Part model, mm, in its own coordinate system. Face numbers are marked on the shaded views. Give positions to 0.01 mm unless a question says otherwise; leave off trailing zeros. Write each loop counter-clockwise with the first axis right and the second up, starting at its lowest first coordinate (ties: lowest second). Pieces come first, ordered by that corner, then holes. Notation, with made-up numbers: M 72,-37.5 L 82,-37.5 A9 ccw 82,-26.5 Z; hole C 6,-25 d5. An arc over 180 degrees is marked long. Write item = value, one per line. Start each with the question number.
from build123d import *

# Parameters (mm, degrees)
F1_DEPTH = 12.7
F2_D     = 19.05
F3_D     = 9


with BuildPart() as f1:
    # F0 (on Top) → F1 (new body)
    with BuildSketch(Plane.XY):
        with BuildLine():
            Line((5.9523138316, 18.7402282516), (-1.5792061086, 25.3897088273))
            Line((-1.5792061086, 25.3897088273), (-8.2286866843, 17.858188887))
            ThreePointArc((-8.2286866843, 17.858188887), (-7.5315199403, 6.6494805757), (-18.7402282516, 5.9523138316))
            Line((-18.7402282516, 5.9523138316), (-25.3897088273, -1.5792061086))
            Line((-25.3897088273, -1.5792061086), (-17.858188887, -8.2286866843))
            ThreePointArc((-17.858188887, -8.2286866843), (-6.6494805757, -7.5315199403), (-5.9523138316, -18.7402282516))
            Line((-5.9523138316, -18.7402282516), (1.5792061086, -25.3897088273))
            Line((1.5792061086, -25.3897088273), (8.2286866843, -17.858188887))
            ThreePointArc((8.2286866843, -17.858188887), (7.5315199403, -6.6494805757), (18.7402282516, -5.9523138316))
            Line((18.7402282516, -5.9523138316), (25.3897088273, 1.5792061086))
            Line((25.3897088273, 1.5792061086), (17.858188887, 8.2286866843))
            ThreePointArc((17.858188887, 8.2286866843), (6.6494805757, 7.5315199403), (5.9523138316, 18.7402282516))
        make_face()
    extrude(amount=F1_DEPTH)

    # F2 (through all)
    with Locations(Plane(origin=(0, 0, 0), x_dir=(1, 0, 0), z_dir=(0, 0, -1))):
        with Locations((0, 0)):
            Hole(F2_D / 2)

    # F3 (through all)
    with Locations(Plane(origin=(0, 0, 0), x_dir=(1, 0, 0), z_dir=(0, 0, -1))):
        with Locations((18.2992085693, -1.1381864263), (-1.1381864263, -18.2992085693), (-18.2992085693, 1.1381864263), (1.1381864263, 18.2992085693)):
            Hole(F3_D / 2)


solid = f1.part
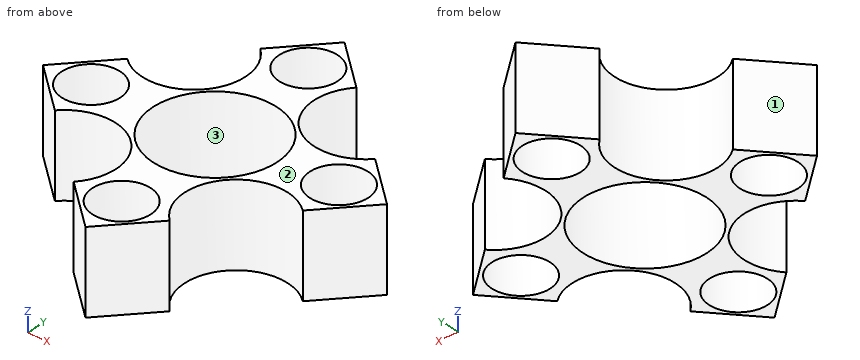
Q1. Probe line 1 along Y through (x, z) = (0, 8.5) (3 decimals); line 2 along X through (y, z) = (7, 6.25); line 3 along Y through (x, z) = (-7.5, 10). List the from-to ranges inside material, lowest first.
Q2. Slice it at D-D (x = 15.5). Give the cut face in (y, z), and give its area (3 significant figures).
Q3. Slice it at B-B (y = 0). Give the cut face in (x, z) (3 decimals), and give its area (3 significant figures).
Q4. Drop flat-ended pins along their axis: P1, Ø8, axis at x = -1.14, y = 18.3, coming from the +Z side; P2, Ø11.5, axis at x = 1.14, y = -18.3, coming from the -Z side; P3, Ø3, axis at y = -13.5, z = 2.5, coming from the +X side; P4, Ø2, axis at y = -9, z = 10, coming from the +X side. Give the stop position or say it passes through.
Q5. Two-plate mould, pull along Y, no slides. Class the marked faces 1, 2 and 3: +Y half, -Y half, draft (parallel to the pull), parting line (faces both ways), or undercut.
Working result:
q1.line_1 = -23.995 to -22.653, -13.946 to -9.525, 9.525 to 13.946, 22.653 to 23.995
q1.line_2 = -7.24 to -6.46, 6.46 to 7.32, 16.49 to 19.25
q1.line_3 = -6.88 to -5.87, 5.87 to 6.69, 17.13 to 18.68
q2.outline = M -4.22,0 L -2.39,0 L -2.39,12.7 L -4.22,12.7 Z; M 4.66,0 L 6.4,0 L 6.4,12.7 L 4.66,12.7 Z
q2.area = 45.5 mm2
q3.outline = M -23.995,0 L -22.653,0 L -22.653,12.7 L -23.995,12.7 Z; M -13.946,0 L -9.525,0 L -9.525,12.7 L -13.946,12.7 Z; M 9.525,0 L 13.946,0 L 13.946,12.7 L 9.525,12.7 Z; M 22.653,0 L 23.995,0 L 23.995,12.7 L 22.653,12.7 Z
q3.area = 146 mm2
q4.P1 = through
q4.P2 = 0
q4.P3 = 6.17
q4.P4 = 6.57
q5.face_1 = +Y half
q5.face_2 = draft
q5.face_3 = undercut
